Input: dimensioned drawing with shaded views. Units: mm. Origin: part minimum x, y, z. A direction names the side the tool comes from. Coordinates: 2 decimals unless noted, no trailing zeros. Order: outer loops, then holes, each group sorted by start corner. A loop starts at its lowest first (then second) coordinate and runs counter-clockwise, first axis right, second up. Notation, with made-up numbers: (12.5, 0) - (63.5, 0) arc R18 cw to (63.5, 29) - close; hole circle Ø1 at (5, 24.5). An arc over 180 degrees is marked (long way). One line per question, with ' | ' between items. Start each with the question number.
(1) Access query for the marked faces 4 and 5. Directions: +Z, -Z, +X, -X, +Y, -Y. A direction counts if a zero-diameter tool reaches every point of the face in a straight line with its end or side. Return the directions, or none.
(2) Line query: line 1 along Z through (x, y) = (9.75, 11) (1 decimal); line 2 along Z through (x, y) = (8, 9.5); line 3 along X through (y, z) = (4.6, 9). Output: solid intervals per line, ascending.
(3) Section C-C (x = 14.75). Return the cut outline in (y, z), then the cut area to 3 significant figures.
(4) Section A-A (y = 9). Return the cut outline in (x, z), then the cut area to 3 significant figures.
(5) Section D-D (y = 7). Return the cut outline in (x, z) (3 decimals).
(6) Draft query along Y for the marked faces 1, 2 and 3. Return one class per face: +Y half, -Y half, draft (parallel to the pull), parting line (faces both ways), or undercut.
(7) Section B-B (z = 9). Return the cut outline in (x, y).
(8) Contact query for flat-ended pins moving along their axis: P1, Ø3, axis at x = 17, y = 10.5, coming from the +Z side; P2, Ø5.5, axis at y = 10.5, z = 28, coming from the +X side; P3, Ø9, axis at y = 9.5, z = 26, coming from the -X side. Output: stop coordinate, or through.
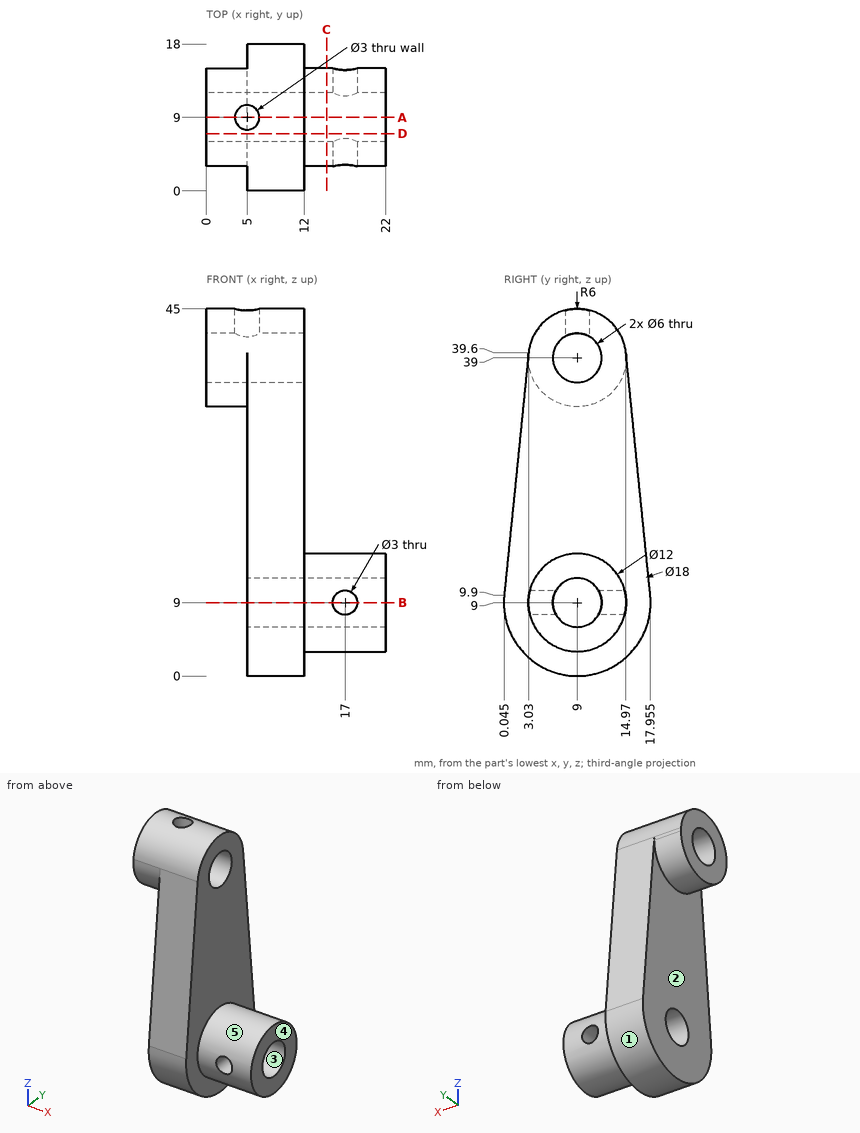
Response values:
1) face 4: +Z, -Z, +X, +Y, -Y | face 5: +X
2) line 1: z = 0.2 to 6.8, 11.2 to 36.8, 41.2 to 44.7 | line 2: z = 0.01 to 6.04, 11.96 to 36.04, 41.96 to 44.98 | line 3: x = 5 to 15.5, 18.5 to 22
3) outline: circle Ø12 at (9, 9); hole circle Ø6 at (9, 9) | area: 84.8 mm²
4) outline: (0, 33) - (5, 33) - (5, 12) - (22, 12) - (22, 15) - (12, 15) - (12, 36) - (0, 36) - close; (0, 42) - (3.5, 42) - (3.5, 45) - (0, 45) - close; (5, 0) - (12, 0) - (12, 3) - (22, 3) - (22, 6) - (5, 6) - close; (6.5, 42) - (12, 42) - (12, 45) - (6.5, 45) - close | area: 312 mm²
5) outline: (0, 33.343) - (5, 33.343) - (5, 11.236) - (22, 11.236) - (22, 14.657) - (12, 14.657) - (12, 36.764) - (0, 36.764) - close; (0, 41.236) - (12, 41.236) - (12, 44.657) - (0, 44.657) - close; (5, 0.225) - (12, 0.225) - (12, 3.343) - (22, 3.343) - (22, 6.764) - (5, 6.764) - close
6) face 1: parting line | face 2: draft | face 3: undercut
7) outline: (5, 0) - (12, 0) - (12, 3) - (15.5, 3) - (15.5, 6) - (5, 6) - close; (5, 12) - (15.5, 12) - (15.5, 15) - (12, 15) - (12, 18) - (5, 18) - close; (18.5, 3) - (22, 3) - (22, 6) - (18.5, 6) - close; (18.5, 12) - (22, 12) - (22, 15) - (18.5, 15) - close
8) P1: stops at z = 15 | P2: stops at x = 12 | P3: stops at x = 5
